Check sheet for the modelled part. Datum: model origin and axes. Units: mm. Give positions to 0.01 mm unless a question says otherwise; leave off trailing zeros. Write each loop counter-clockwise with the first axis right and the second up, starting at its lowest first coordinate (ties: lowest second). Pieces come first, ordered by that corner, then holes. Notation, with made-up numbers: M 49,30.25 L 88,30.25 A30 ccw 88,68.25 Z; hole C 70.5,-21 d9. An arc over 180 degrees is marked long. Write each question's results on one line, items separated by ' | '. Start each with the question number.
Solid Edge part; units mm, degrees
sketch "Sketch1" plane through (0, 0, 0) normal (0, -1, 0) x (1, 0, 0)
  line L0 (4, 0) -> (1.8, 0)
  line L1 (1.8, 0) -> (1.8, -1.4)
  line L2 (1.8, -1.4) -> (2, -1.4)
  line L3 (2, -1.4) -> (2, -50)
  line L4 (2, -50) -> (0, -50)
  arc A0 (0, 3.1) -> (4, 2.0282) centre (0, -4.9) cw
  line L5 (4, 0) -> (4, 2.0282)
  dimension "D1" = 1.8
  dimension "D2" = 1.8
revolve "RevolvedProtrusion1" add sketch "Sketch1" angle 360 about axis through (0, 0, -6) along (0, 0, 1)
cosmetic_thread "Thread1"
chamfer "Chamfer_1" distance 0.4 angle 45 1 edges at (-2, 0, -50)
fillet "Round1" radius 0.2 2 edges at (-1.8, 0, -1.4) (-1.8, 0, 0)
fillet "Round_3" radius 1 1 edges at (-4, 0, 2.0282)
sketch "Sketch2" plane through (0, 0, 3.1) normal (0, 0, 1) x (1, 0, 0)
  line L0 (-0.5, 0.5) -> (-0.5, 2.3)
  line L1 (-0.5, 2.3) -> (0.5, 2.3)
  line L2 (0.5, 2.3) -> (0.5, 0.5)
  line L3 (0.5, 0.5) -> (2.3, 0.5)
  line L4 (2.3, 0.5) -> (2.3, -0.5)
  line L5 (2.3, -0.5) -> (0.5, -0.5)
  line L6 (0.5, -0.5) -> (0.5, -2.3)
  line L7 (0.5, -2.3) -> (-0.5, -2.3)
  line L8 (-0.5, -2.3) -> (-0.5, -0.5)
  line L9 (-0.5, -0.5) -> (-2.3, -0.5)
  line L10 (-2.3, -0.5) -> (-2.3, 0.5)
  line L11 (-2.3, 0.5) -> (-0.5, 0.5)
  dimension "D1" = 0.5
extrude "ExtrudedCutout_2" cut sketch "Sketch2" against normal blind 2.3
properties part number "STD-DIN_7985-M4x50" material "Galvanized steel"
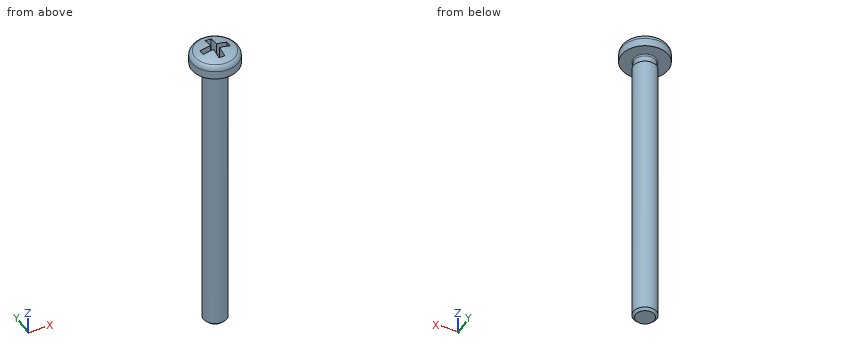
Q1. Depth check by flat-ended pin: pin 1 Ø0.8 at (x, z) = (0, 2) entering from -Y; pin 2 Ø4 at (y, z) = (-0.5, -22.5) entering from +X; pin 3 Ø1.4 at (x, z) = (-1.5, 2.5) entering from -Y. Enter the tip coordinate at first touch or a pass-through.
Q2. Section check A-A on z = -4. Record the boundary of the cut face in (x, y), plus the area to 3 significant figures.
Q3. Scan lines: L1, parallel to Z at x = 3.5, y = 0; L2, parallel to X at y = 1.5, z = 1.5; L3, parallel to Z at x = -0.5, y = 3.75. Record each from-to range of solid material in increasing order.
Check result:
1) pin 1: y = -3.98 | pin 2: x = 2 | pin 3: y = -3.71
2) outline: C 0,0 d4 | area: 12.6 mm^2
3) L1: 0 to 2.29 | L2: -3.71 to -0.5, 0.5 to 3.71 | L3: 0 to 2.05
